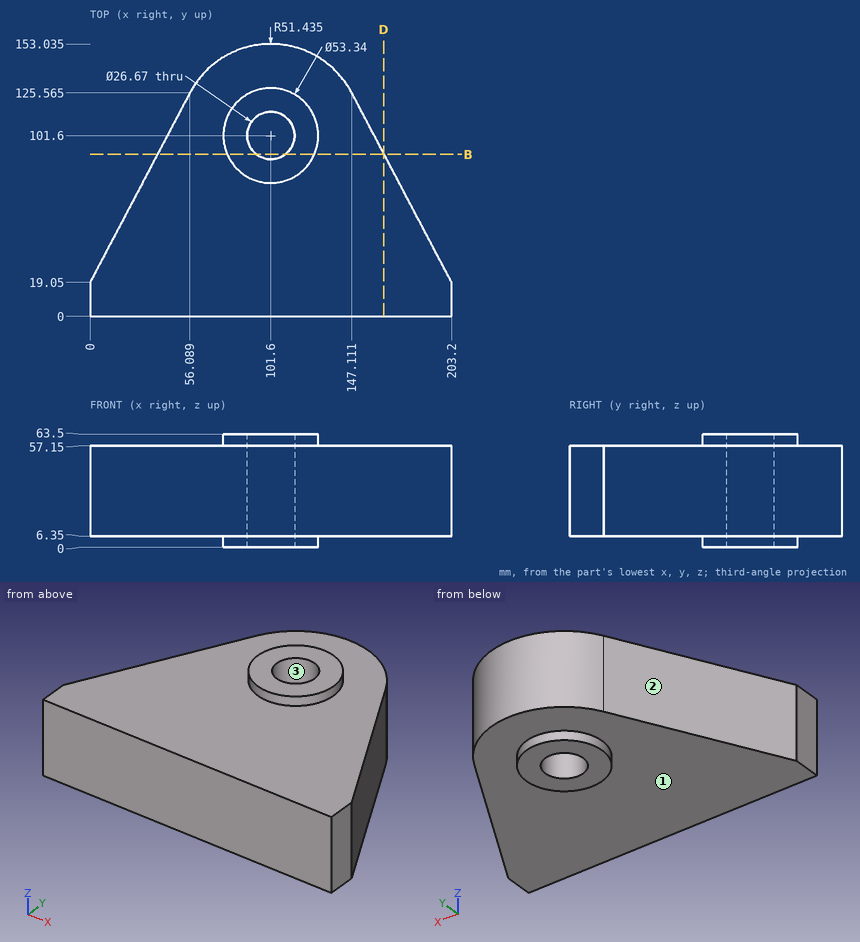
Could you check a few things on this drawing? It's one solid part, dimensions in mm from its lowest x, y, z. Coordinates: 2 decimals unless noted, no trailing zeros. Order: outer loops, then holes, each group sorted by start corner. A loop starts at its lowest first (then second) coordinate and runs counter-clockwise, first axis right, second up. Notation, with made-up numbers: M 0,48 L 52,48 A19 cw 52,83 Z; hole C -6.5,-11.75 d9. An arc over 180 degrees is marked long. Use one line per item in the form item = value. Start each with the question number.
1. For pin 1 (12 mm diameter, centred on y = 61.5, z = 34.5, fed in from -X); pin 2 (4 mm diameter, centred on x = 53, y = 95, fed in from +Z); pin 3 (2 mm diameter, centred on y = 98.5, z = 40.5, fed in from +X), each with a flat end and sliding along its axis, tell me the tip position at first contact or that it passes through.
2. Suppose I cut it at B-B on y = 91. Write out the boundary of the cut face in (x, z), then the cut area to 3 significant figures.
3. Suppose I cut it at D-D on x = 165. Write out the boundary of the cut face in (y, z).
4. We'd pull the mould along Y, two halves only. Please class the marked faces 1, 2 and 3: +Y half, -Y half, draft (parallel to the pull), parting line (faces both ways), or undercut.
5. Please list where these lines run through material, in increasing order: line 1 (Y direction, x = 101.6, z = 26) (1 decimal); line 2 (Z direction, x = 148.5, y = 118); line 3 (X direction, y = 101.6, z = 24) (1 decimal).
Geometry says:
q1.pin_1 = 19.19
q1.pin_2 = 57.15
q1.pin_3 = 161.89
q2.outline = M 37.89,6.35 L 77.13,6.35 L 77.13,0 L 93.51,0 L 93.51,63.5 L 77.13,63.5 L 77.13,57.15 L 37.89,57.15 Z; M 109.69,0 L 126.07,0 L 126.07,6.35 L 165.31,6.35 L 165.31,57.15 L 126.07,57.15 L 126.07,63.5 L 109.69,63.5 Z
q2.area = 6,070 mm^2
q3.outline = M 0,6.35 L 91.59,6.35 L 91.59,57.15 L 0,57.15 Z
q4.face_1 = draft
q4.face_2 = +Y half
q4.face_3 = undercut
q5.line_1 = 0 to 88.3, 114.9 to 153
q5.line_2 = 6.35 to 57.15
q5.line_3 = 43.5 to 88.3, 114.9 to 159.7
